Work out the finished part from the listing and answer in its coordinate system (mm). A direction names the side the tool comes from. Round coordinates to 2 decimals unless told otherwise and drop trailing zeros. Loops run counter-clockwise (first coordinate to the right, second up) from the corner with the lowest first, then second, coordinate; pieces in that order, holes last. Notation, with made-up numbers: (-34, 68) - (20, 68) arc R16 ccw to (20, 93) - close; hole circle Ø9 at (87.5, 83). An arc over 180 degrees is marked (long way). Return JSON: item names as keys, results as strings.
from build123d import *

# Parameters (mm, degrees)
F0_R           = 1.65
F1_DEPTH       = 17
F2_DEPTH       = 8
F3_DEPTH       = 5
F6_D           = 4
F6_CSINK_D     = 8.7
F6_CSINK_ANGLE = 90


with BuildPart() as f1:
    # F0 (on Front) → F1 (new body)
    with BuildSketch(Plane.XZ):
        Polygon((10, 25), (0, 25), (-10, 25), (-17.5, 25), (-17.5, 0), (-17.5, -25), (-10, -25), (0, -25), (10, -25), (17.5, -25), (17.5, 25), align=None)
        with BuildLine():
            ThreePointArc((0, 15), (10.606602, 10.606602), (15, 0))
            ThreePointArc((15, 0), (-10.606602, -10.606602), (0, 15))
        make_face(mode=Mode.SUBTRACT)
        with BuildLine():
            ThreePointArc((0, 15), (-10.606602, -10.606602), (15, 0))
            ThreePointArc((15, 0), (10.606602, 10.606602), (0, 15))
        make_face()
        Circle(F0_R, mode=Mode.SUBTRACT)
        Polygon((-10, 25), (0, 25), (10, 25), (10, 35), (0, 35), (-10, 35), align=None)
        Polygon((10, -35), (10, -25), (0, -25), (-10, -25), (-10, -35), (0, -35), align=None)
    extrude(amount=F1_DEPTH)

    # F0 (on Front) → F2 (cut)
    with BuildSketch(Plane.XZ):
        with BuildLine():
            ThreePointArc((0, 15), (-10.606602, -10.606602), (15, 0))
            ThreePointArc((15, 0), (10.606602, 10.606602), (0, 15))
        make_face()
        Circle(F0_R, mode=Mode.SUBTRACT)
    extrude(amount=F2_DEPTH, mode=Mode.SUBTRACT)

    # F0 (on Front) → F3 (cut)
    with BuildSketch(Plane.XZ):
        Polygon((-10, 25), (0, 25), (10, 25), (10, 35), (0, 35), (-10, 35), align=None)
        Polygon((10, -35), (10, -25), (0, -25), (-10, -25), (-10, -35), (0, -35), align=None)
    extrude(amount=F3_DEPTH, mode=Mode.SUBTRACT)

    # F6 (through all)
    with Locations(Plane(origin=(0, -5, 0), x_dir=(-1, 0, 0), z_dir=(0, 1, 0))):
        with Locations((0, -30), (0, 30)):
            CounterSinkHole(F6_D / 2, F6_CSINK_D / 2, counter_sink_angle=F6_CSINK_ANGLE)


solid = f1.part
1) Section A-A (z = 30) is taken. Give the vertices of the cut face in (x, y).
Verdict:
{"outline": "(-10, -17) - (-2, -17) - (-2, -7.35) - (-4.35, -5) - (-10, -5) - close; (2, -17) - (10, -17) - (10, -5) - (4.35, -5) - (2, -7.35) - close"}
2) A tool of negligible diameter and unlimited length cuts with its end or side. For faces 5 (the flat face through (10, -11, 30)), 6 (the flat face through (0, -8, -3)), 7 (the flat face through (-10, -11, 30)), from which of +Z, -Z, +X, -X, +Y, -Y can it reach the whole face along a straight path? Write none if from no direction.
Verdict:
{"face 5": "+Z, +X, +Y, -Y", "face 6": "+Y", "face 7": "+Z, -X, +Y, -Y"}
3) Section B-B (y = -14.5) is taken. Give the vertices of the cut face in (x, z), and give its area (3 significant figures).
Verdict:
{"outline": "(-17.5, -25) - (-10, -25) - (-10, -35) - (10, -35) - (10, -25) - (17.5, -25) - (17.5, 25) - (10, 25) - (10, 35) - (-10, 35) - (-10, 25) - (-17.5, 25) - close; hole circle Ø4 at (0, -30); hole circle Ø4 at (0, 30); hole circle Ø3.3 at (0, 0)", "area": "2,120 mm2"}
4) Section D-D (z = -14) is taken. Give the vertices of the cut face in (x, y).
Verdict:
{"outline": "(-17.5, -17) - (17.5, -17) - (17.5, 0) - (5.39, 0) - (5.39, -8) - (-5.39, -8) - (-5.39, 0) - (-17.5, 0) - close"}
5) Section C-C (x = -11) is taken. Give the vertices of the cut face in (y, z).
Verdict:
{"outline": "(-17, -25) - (0, -25) - (0, -10.2) - (-8, -10.2) - (-8, 10.2) - (0, 10.2) - (0, 25) - (-17, 25) - close"}
6) Determine the mould class of faces 1 (the flat face through (17.5, -8, 0)), 2 (the conical face through (-0.46, -7.24, 27.94)), 3 (the cylindrical face through (0, -12, 28)), 4 (the flat face through (-0.2, -4.6, -25)) for opening direction Z: pulls with the +Z half, pulls with the -Z half, needs draft (parallel to the pull), parting line crosses it, or undercut.
Verdict:
{"face 1": "needs draft", "face 2": "undercut", "face 3": "undercut", "face 4": "pulls with the -Z half"}
7) Flat-ended cylindrical pins translate along their axes: pin 1 (15 mm diameter, centred on x = -0.5, z = 2, fed in from +Y); pin 2 (3 mm diameter, centred on y = -10, z = 28, fed in from +X); pin 3 (3 mm diameter, centred on x = 3.5, z = -32.5, fed in from +Y). Find the tip coordinate at first contact, or state that the pin passes through.
Verdict:
{"pin 1": "stops at y = -8", "pin 2": "stops at x = 10", "pin 3": "stops at y = -5"}
8) Find the intervals of material crossed by L1, parallel to Z at x = 0, y = -11; L2, parallel to X at y = -10.5, z = 30; L3, parallel to Z at x = -14, y = -9.5, in increasing order.
Verdict:
{"L1": "z = -35 to -32, -28 to -1.65, 1.65 to 28, 32 to 35", "L2": "x = -10 to -2, 2 to 10", "L3": "z = -25 to 25"}
